from build123d import *

# Parameters (mm, degrees)
F0_W     = 900
F0_H     = 140
F1_DEPTH = 70
F2_R     = 10
F4_DEPTH = 20


with BuildPart() as f1:
    # F0 (on Front) → F1 (new body)
    with BuildSketch(Plane.XZ):
        Rectangle(F0_W, F0_H)
    extrude(amount=F1_DEPTH)

    # F2
    f2_edges = [f1.edges().sort_by_distance(p)[0] for p in [
        (0, -70, 70),
        (0, 0, 70),
        (0, -70, -70),
        (0, 0, -70),
    ]]
    fillet(f2_edges, radius=F2_R)

    # F3 (on face) → F4 (join)
    with BuildSketch(Plane(origin=(0, 0, 0), x_dir=(-1, 0, 0), z_dir=(0, 1, 0))):
        with BuildLine():
            ThreePointArc((375, 30), (369.142136, 44.142136), (355, 50))
            Line((355, 50), (-355, 50))
            ThreePointArc((-355, 50), (-369.142136, 44.142136), (-375, 30))
            Line((-375, 30), (-375, -30))
            ThreePointArc((-375, -30), (-369.142136, -44.142136), (-355, -50))
            Line((-355, -50), (355, -50))
            ThreePointArc((355, -50), (369.142136, -44.142136), (375, -30))
            Line((375, -30), (375, 30))
        make_face()
    extrude(amount=F4_DEPTH)


solid = f1.part
Input: part model. Units: mm. Frame: model coordinates. A direction names the side the tool comes from. Give positions to 0.01 mm unless a question says otherwise; leave off trailing zeros. Order: outer loops, then holes, each group sorted by start corner. A loop starts at its lowest first (then second) coordinate and runs counter-clockwise, first axis right, second up. Notation, with made-up numbers: (11, -29.75) - (49, -29.75) arc R13 ccw to (49, -8.75) - close; hole circle Ø11 at (-19, -17.75). An arc over 180 degrees is marked (long way). Answer as a JSON object with one key per item and string values. Group by question number.
Q1. Line query: probe 1 along Y at (x, z) = (183.5, 60.5); probe 2 along X at (y, z) = (4, 29.5); probe 3 along Z at (x, y) = (-8, 6.5). Output: solid intervals per line, ascending.
Q2. Cut plane B-B, the plane z = -1.5. Output: boundary loops of the cut face in (x, y), then the cut area to 3 significant figures.
Q3. First-contact query: pin 1 Ø12 at (x, y) = (-3.5, 1) entering from +Z; pin 2 Ø6 at (x, y) = (-70, 6.5) entering from -Z; pin 3 Ø10 at (y, z) = (8.5, -8.5) entering from +X. Flat tips, straight axial feed; report the tip coordinate or a pass-through.
Q4. Set-up query: faces 1 (the face through (369.297, 9.86, -43.986)), 2 (the face through (-369.297, 9.86, 43.986)), 3 (the face through (-368.986, 9.86, -44.297)), 4 (the face through (5, 10, -50)), 5 (the face through (375, 10, 0)). Return all of +Z, -Z, +X, -X, +Y, -Y with unobstructed straight access to the full face (end or side cutting, diameter ignored); none if empty.
Q5. Cut plane C-C, the plane y = 10. Output: boundary loops of the cut face in (x, z).
Q6. Cut plane A-A, the plane x = -81. Output: boundary loops of the cut face in (y, z).
Results:
{
 "1": {"probe 1": "-69.99 to -0.01", "probe 2": "-375 to 375", "probe 3": "-50 to 50"},
 "2": {"outline": "(-450, -70) - (450, -70) - (450, 0) - (375, 0) - (375, 20) - (-375, 20) - (-375, 0) - (-450, 0) - close", "area": "78,000 mm^2"},
 "3": {"pin 1": "z = 68.66", "pin 2": "z = -50", "pin 3": "x = 375"},
 "4": {"face 1": "-Z, +X, +Y", "face 2": "+Z, -X, +Y", "face 3": "-Z, -X, +Y", "face 4": "-Z, +X, -X, +Y", "face 5": "+Z, -Z, +X, +Y"},
 "5": {"outline": "(-375, -30) arc R20 ccw to (-355, -50) - (355, -50) arc R20 ccw to (375, -30) - (375, 30) arc R20 ccw to (355, 50) - (-355, 50) arc R20 ccw to (-375, 30) - close"},
 "6": {"outline": "(-70, -60) arc R10 ccw to (-60, -70) - (-10, -70) arc R10 ccw to (0, -60) - (0, -50) - (20, -50) - (20, 50) - (0, 50) - (0, 60) arc R10 ccw to (-10, 70) - (-60, 70) arc R10 ccw to (-70, 60) - close"}
}
